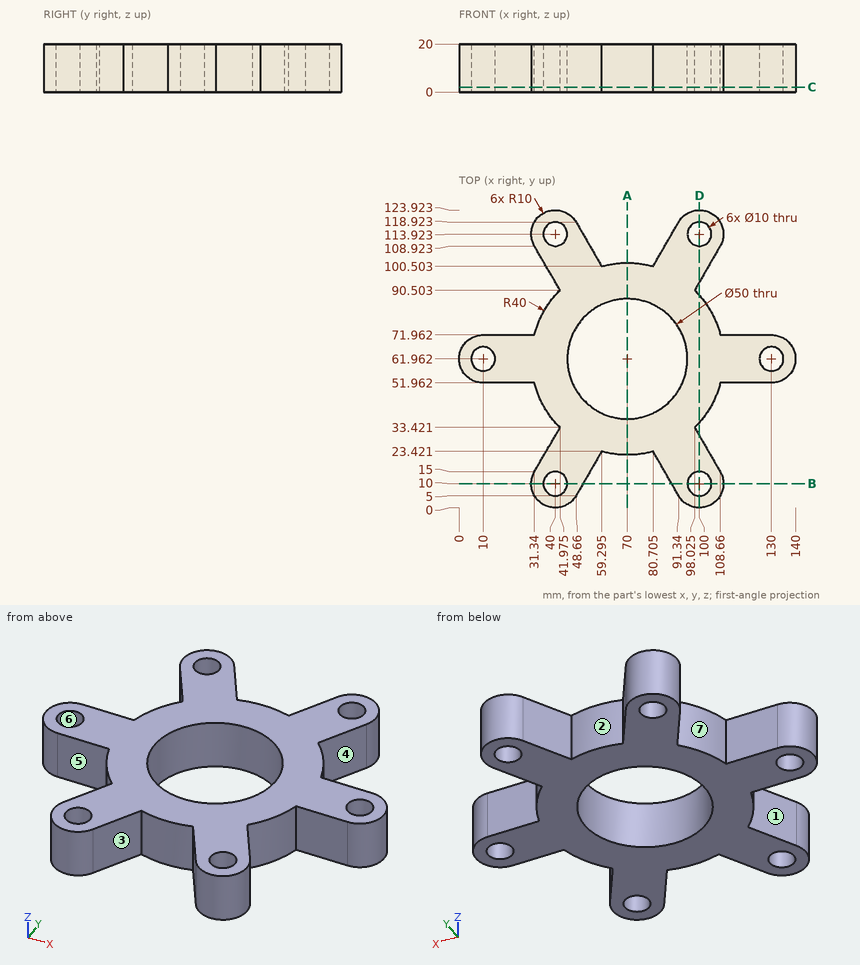
Input: dimensioned drawing with shaded views. Units: mm. Origin: part minimum x, y, z. A direction names the side the tool comes from. Give positions to 0.01 mm unless a question says otherwise; leave off trailing zeros. Write each loop counter-clockwise with the first axis right and the second up, starting at its lowest first coordinate (ties: lowest second). Pieces come first, ordered by that corner, then holes.
Q1. Material intervals for probe 1 along Y at (x, z) = (130, 11.5); probe 2 along Y at (x, z) = (100, 8) (1 decimal); probe 3 along X at (y, z) = (110, 5.75) (1 decimal), sorted ascending.
Q2. Section C-C, the plane z = 2. State how many separate pieces and enclosed holes the cut face has.
Q3. Pull-direction query (X, two-part tool) for the marked faces 5, 6 and 7; classes: pulls with the +X half, pulls with the -X half, needs draft (parallel to the pull), parting line crosses it, or undercut.
Q4. Section A-A, the plane x = 70. Output: boundary loops of the cut face in (y, z).
Q5. Section D-D, the plane x = 100. Output: boundary loops of the cut face in (y, z) (1 decimal), plus the area to 3 significant figures.
Q6. First-contact query: P1, Ø10, axis at x = 91, z = 15.5, coming from the -Y side (1 decimal); P2, Ø4, axis at y = 38.5, z = 8.5, coming from the +X side (1 decimal); P3, Ø6, axis at x = 10, y = 61.96, coming from the -Z side; P4, Ø10, axis at x = 124.5, z = 14, coming from the -Y side. Flat tips, straight axial feed; report the tip coordinate or a pass-through.
Q7. Section B-B, the plane y = 10. Output: boundary loops of the cut face in (x, z), plus the area to 3 significant figures.
Q8. Set-up query: the marked faces 1, 2, 3 and 4. Return all of +Z, -Z, +X, -X, +Y, -Y with unobstructed straight access to the full face (end or side cutting, diameter ignored); none if empty.
Filled in:
1. probe 1: y = 51.96 to 56.96, 66.96 to 71.96
1. probe 2: y = 0 to 5, 15 to 30, 35.5 to 88.4, 93.9 to 108.9, 118.9 to 123.9
1. probe 3: x = 30.8 to 36.9, 43.1 to 53.8, 86.2 to 96.9, 103.1 to 109.2
2. separate pieces: 1
2. enclosed holes: 7
3. face 5: needs draft
3. face 6: undercut
3. face 7: pulls with the -X half
4. outline: (21.96, 0) - (36.96, 0) - (36.96, 20) - (21.96, 20) - close; (86.96, 0) - (101.96, 0) - (101.96, 20) - (86.96, 20) - close
5. outline: (0, 0) - (5, 0) - (5, 20) - (0, 20) - close; (15, 0) - (30, 0) - (30, 20) - (15, 20) - close; (35.5, 0) - (88.4, 0) - (88.4, 20) - (35.5, 20) - close; (93.9, 0) - (108.9, 0) - (108.9, 20) - (93.9, 20) - close; (118.9, 0) - (123.9, 0) - (123.9, 20) - (118.9, 20) - close
5. area: 1,860 mm2
6. P1: stops at y = 0.8
6. P2: stops at x = 103.8
6. P3: passes through
6. P4: stops at y = 51.96
7. outline: (30, 0) - (35, 0) - (35, 20) - (30, 20) - close; (45, 0) - (51.55, 0) - (51.55, 20) - (45, 20) - close; (88.45, 0) - (95, 0) - (95, 20) - (88.45, 20) - close; (105, 0) - (110, 0) - (110, 20) - (105, 20) - close
7. area: 462 mm2
8. face 1: +Z, -Z, -X
8. face 2: +Z, -Z, +Y
8. face 3: +Z, -Z, -Y
8. face 4: +Z, -Z, +X
